Answer from the drawing. Dimensions are ordinates in mm from the lowest x, y and z of the part. A direction names the side the tool comes from. Give positions to 0.01 mm unless a question says otherwise; leave off trailing zeros. Order: outer loops, then holes, each group sorted by start corner. A loop starts at its lowest first (then second) coordinate and runs counter-clockwise, first axis right, second up. Notation, with made-up numbers: (71.25, 86) -> (77.25, 86) arc R15 ccw to (77.25, 103) -> close; hole circle Ø11 at (18.5, 54). An arc over 180 degrees is marked (long way). One line per question, with ' | ' between items. Start each with the question number.
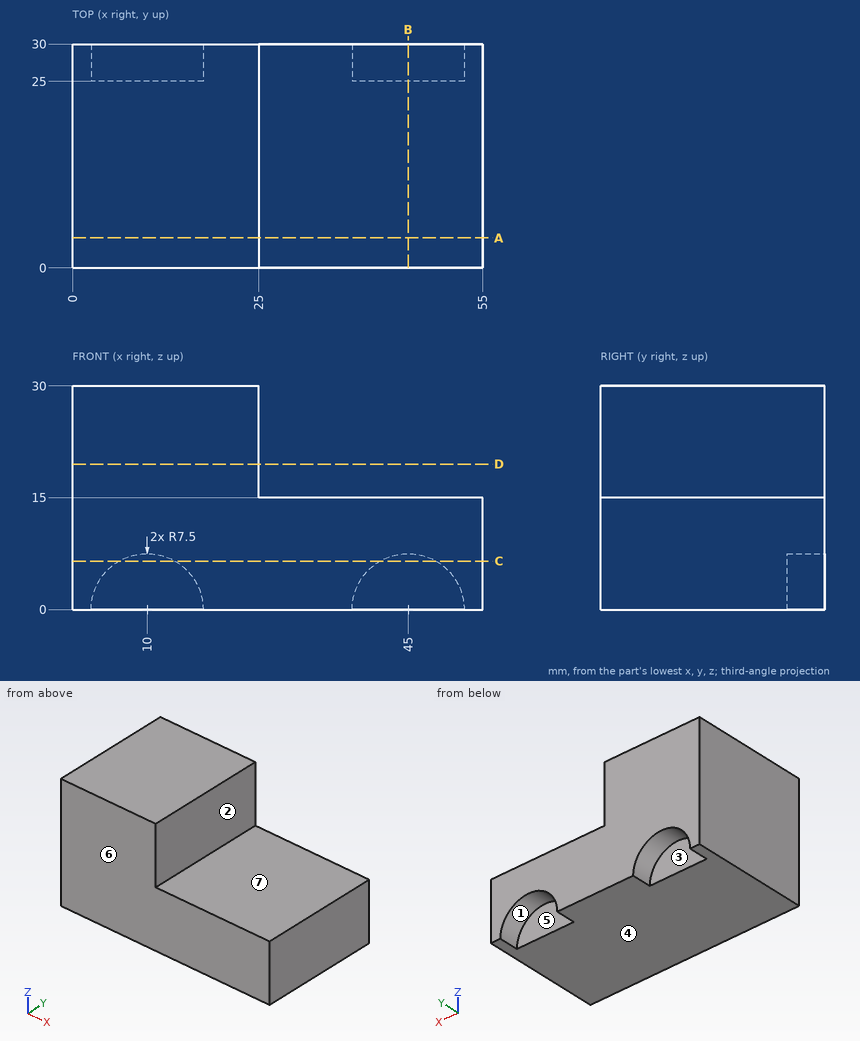
(1) The part is cut by section C-C on z = 6.5. Determine the outline of the cut face in (x, y), plus the area to 3 significant figures.
(2) Given P1, Ø6, axis at y = 8, z = 26, coming from the -X side; P2, Ø4, axis at x = 7, z = 2, coming from the +Y side; P3, Ø7.5, axis at y = 16, z = 24.5, coming from the +X side; P4, Ø5, axis at x = 48.5, y = 23, coming from the +Z side, each flat-ended and moving along its own axis, determine where each tip first touches the part or whether it passes through.
(3) Consider line 1 (X direction, y = 28.5, z = 6.25); line 2 (Z direction, x = 31.5, y = 10.5); line 3 (X direction, y = 14, z = 21.75). Determine where each line is inside the solid, lowest interval first.
(4) The part is cut by section B-B on x = 45. Determine the outline of the cut face in (y, z).
(5) The part is cut by section A-A on y = 4. Determine the outline of the cut face in (x, z).
(6) Determine the mould class of the marked faces 1, 2, 3 and 4 for opening direction X: pulls with the +X half, pulls with the -X half, needs draft (parallel to the pull), parting line crosses it, or undercut.
(7) The part is cut by section D-D on z = 19.5. Determine the outline of the cut face in (x, y).
(8) For the marked faces 5, 6 and 7, determine the directions among +Z, -Z, +X, -X, +Y, -Y from which every point of the face is accessible in a straight line to the end or side of a thin tool.
Result sheet:
1) outline: (0, 0) -> (55, 0) -> (55, 30) -> (48.74, 30) -> (48.74, 25) -> (41.26, 25) -> (41.26, 30) -> (13.74, 30) -> (13.74, 25) -> (6.26, 25) -> (6.26, 30) -> (0, 30) -> close | area: 1,580 mm^2
2) P1: stops at x = 0 | P2: stops at y = 25 | P3: stops at x = 25 | P4: stops at z = 15
3) line 1: x = 0 to 5.85, 14.15 to 40.85, 49.15 to 55 | line 2: z = 0 to 15 | line 3: x = 0 to 25
4) outline: (0, 0) -> (25, 0) -> (25, 7.5) -> (30, 7.5) -> (30, 15) -> (0, 15) -> close
5) outline: (0, 0) -> (55, 0) -> (55, 15) -> (25, 15) -> (25, 30) -> (0, 30) -> close
6) face 1: undercut | face 2: pulls with the +X half | face 3: undercut | face 4: needs draft
7) outline: (0, 0) -> (25, 0) -> (25, 30) -> (0, 30) -> close
8) face 5: -Z, +Y | face 6: +Z, -Z, +X, -X, -Y | face 7: +Z, +X, +Y, -Y
